from build123d import *

# Parameters (mm, degrees)
SKETCH_1_R      = 2
EXTRUDE_2_DEPTH = 2
FILLET_1_R      = 5


with BuildPart() as part:
    # 草图1 → 凸台-拉伸2 (new body)
    with BuildSketch(Plane.XY):
        with BuildLine():
            Line((3.5, 32), (3.5, 0))
            ThreePointArc((3.5, 0), (0, -3.5), (-3.5, 0))
            Line((-3.5, 0), (-3.5, 18))
            ThreePointArc((-3.5, 18), (-4.706147584, 24.840402867), (-8.179111138, 30.855752194))
            Line((-8.179111138, 30.855752194), (-9.058182296, 48.949169661))
            ThreePointArc((-9.058182296, 48.949169661), (-6.193568214, 52.5616192), (-2.233608092, 50.200576774))
            Line((-2.233608092, 50.200576774), (3.328697807, 33.08155948))
            ThreePointArc((3.328697807, 33.08155948), (3.456909192, 32.547520628), (3.5, 32))
        make_face()
        with Locations((0, 32)):
            Circle(SKETCH_1_R, mode=Mode.SUBTRACT)
        Circle(SKETCH_1_R, mode=Mode.SUBTRACT)
        with Locations((-5.562305899, 49.119017293)):
            Circle(SKETCH_1_R, mode=Mode.SUBTRACT)
        with BuildLine():
            Line((-6.146357487, 43.946342838), (-5.894516621, 36.910571396))
            ThreePointArc((-5.894516621, 36.910571396), (-2.956230896, 34.539004156), (-1.02143743, 37.781600094))
            Line((-1.02143743, 37.781600094), (-3.222509972, 44.468960057))
            ThreePointArc((-3.222509972, 44.468960057), (-4.91124893, 45.476597506), (-6.146357487, 43.946342838))
        make_face(mode=Mode.SUBTRACT)
    extrude(amount=EXTRUDE_2_DEPTH)

    # 圆角1
    fillet_1_edges = [part.edges().sort_by_distance(p)[0] for p in [
        (-8.179111138, 30.855752194, 1),
    ]]
    fillet(fillet_1_edges, radius=FILLET_1_R)


solid = part.part
Geometry check sheet. Reference: the model listing, model coordinates, mm. A direction names the side the tool comes from. Round coordinates to 2 decimals unless told otherwise and drop trailing zeros. Loops run counter-clockwise (first coordinate to the right, second up) from the corner with the lowest first, then second, coordinate; pieces in that order, holes last.
Item 1: Mould release check, pull along X, two halves, no side actions. Record for faces 4 (the cylindrical face through (-6.26, 52.55, 0.99)), 5 (the flat face through (-1, 25, 0)), 6 (the flat face through (-2.107, 41.078, 0.986)): pulls with the +X half, pulls with the -X half, needs draft (parallel to the pull), parting line crosses it, or undercut.
Item 2: Cross-section at D-D on y = 8.5. Record the boundary of the cut face in (x, z), then the cut area to 3 significant figures.
Item 3: Gauge pin test, flat ends, axial feed: pin 1 (6.5 mm diameter, centred on x = -5.56, y = 49.12, fed in from -Z); pin 2 (3.5 mm diameter, centred on x = 0, y = 0, fed in from +Z) (3 decimals); pin 3 (1 mm diameter, centred on y = 6, z = 1, fed in from -X). Record the tip position at first contact, or that the pin passes through.
Item 4: Access from +Z, -Z, +X, -X, +Y, -Y to the whole of each face (thin tool, end or side, straight path). Record for faces 1 (the cylindrical face through (-4.88, 45.48, 0.99)), 2 (the flat face through (3.5, 16, 1)), 3 (the flat face through (-3.5, 9, 1)).
Item 5: Cross-section at B-B on z = 1.6. Record the boundary of the cut face in (x, y), then the cut area to 3 significant figures.
Item 6: Cross-section at A-A on x = 0. Record the boundary of the cut face in (y, z), then the cut area to 3 significant figures.
Item 7: Cross-section at C-C on x = -5. Record the boundary of the cut face in (y, z).
Item 8: Thickness scan on line 1 (X direction, y = 13.5, z = 1.3); line 2 (X direction, y = 37, z = 1.1); line 3 (X direction, y = 0.5, z = 0.1). Record the ranges inside material, lowest first.
Answer sheet:
1. face 4: parting line crosses it
1. face 5: needs draft
1. face 6: undercut
2. outline: (-3.5, 0) - (3.5, 0) - (3.5, 2) - (-3.5, 2) - close
2. area: 14.0 mm2
3. pin 1: stops at z = 0
3. pin 2: passes through
3. pin 3: stops at x = -3.5
4. face 1: +Z, -Z
4. face 2: +Z, -Z, +X, +Y, -Y
4. face 3: +Z, -Z, -X, -Y
5. outline: (-9.06, 48.95) - (-8.26, 32.43) arc R5 ccw to (-7.31, 29.74) arc R20 cw to (-3.5, 18) - (-3.5, 0) arc R3.5 ccw to (3.5, 0) - (3.5, 32) arc R3.5 ccw to (3.33, 33.08) - (-2.23, 50.2) arc R3.5 ccw to start; hole circle Ø4 at (-5.56, 49.12); hole (-6.15, 43.95) - (-5.89, 36.91) arc R2.5 ccw (long way) to (-1.02, 37.78) - (-3.22, 44.47) arc R1.5 ccw to start; hole circle Ø4 at (0, 0); hole circle Ø4 at (0, 32)
5. area: 370 mm2
6. outline: (-3.5, 0) - (-2, 0) - (-2, 2) - (-3.5, 2) - close; (2, 0) - (30, 0) - (30, 2) - (2, 2) - close; (34, 0) - (43.33, 0) - (43.33, 2) - (34, 2) - close
6. area: 77.7 mm2
7. outline: (25.6, 0) - (35.08, 0) - (35.08, 2) - (25.6, 2) - close; (45.46, 0) - (47.2, 0) - (47.2, 2) - (45.46, 2) - close; (51.04, 0) - (52.57, 0) - (52.57, 2) - (51.04, 2) - close
8. line 1: x = -3.5 to 3.5
8. line 2: x = -8.48 to -5.9, -0.9 to 2.06
8. line 3: x = -3.5 to -1.94, 1.94 to 3.5
